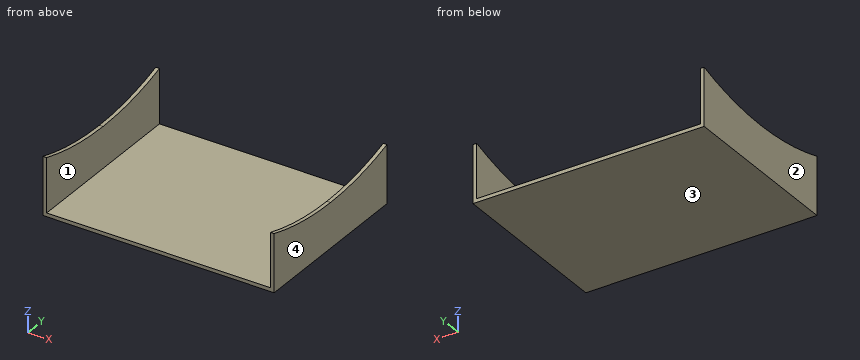
```python
from build123d import *

# Parameters (mm, degrees)
BOSS_EXTRUDE3_DEPTH = 3.18
SKETCH1_5_W         = 3.18
SKETCH1_5_H         = 75
BOSS_EXTRUDE4_DEPTH = 100


with BuildPart() as part:
    # Sketch1 → Boss-Extrude3 (new body)
    with BuildSketch(Plane(origin=(0, 0, 0), x_dir=(0, 0, -1), z_dir=(1, 0, 0))):
        with BuildLine():
            Line((289.494679355, 75), (242.674679355, 75))
            ThreePointArc((242.674679355, 75), (251.152711071, 37.925133117), (254, 0))
            Line((254, 0), (289.494679355, 0))
            Line((289.494679355, 0), (289.494679355, 75))
        make_face()
        with BuildLine():
            Line((289.494679355, 0), (254, 0))
            ThreePointArc((254, 0), (251.152711071, -37.925133117), (242.674679355, -75))
            Line((242.674679355, -75), (289.494679355, -75))
            Line((289.494679355, -75), (289.494679355, 0))
        make_face()
    extrude(amount=BOSS_EXTRUDE3_DEPTH)

    # Sketch1_5 → Boss-Extrude4 (add)
    with BuildSketch(Plane(origin=(0, 0, 0), x_dir=(0, 0, -1), z_dir=(1, 0, 0))):
        with Locations((291.084679355, 37.5)):
            Rectangle(SKETCH1_5_W, SKETCH1_5_H)
        with Locations((291.084679355, -37.5)):
            Rectangle(SKETCH1_5_W, SKETCH1_5_H)
    extrude(amount=BOSS_EXTRUDE4_DEPTH)

    # Mirror2: part across plane


with BuildPart() as part_1:
    add(part.part)
    add(part.part.mirror(Plane(origin=(100, 0, 0), x_dir=(0, 0, 1), z_dir=(1, 0, 0))))


solid = part_1.part
```
Design review of the part built by this model. Coordinates are the model's own, in mm. Face numbers are marked on the shaded views. Round coordinates to 2 decimals unless told otherwise and drop trailing zeros. Order: outer loops, then holes, each group sorted by start corner. A loop starts at its lowest first (then second) coordinate and runs counter-clockwise, first axis right, second up. Notation, with made-up numbers: M 77.25,56 L 82.25,56 A19 ccw 82.25,75 Z; hole C 38.25,-23 d9. An arc over 180 degrees is marked long. Put each result on its own line as item: value.
Q1. Consider section C-C (y = -22). State the section outline as (x, z) points, and give its area (3 significant figures).
Reported:
outline: M 0,-292.67 L 200,-292.67 L 200,-253.05 L 196.82,-253.05 L 196.82,-289.49 L 3.18,-289.49 L 3.18,-253.05 L 0,-253.05 Z
area: 868 mm²
Q2. Consider section D-D (x = 87). State the section outline as (y, z) points, and give its area (3 significant figures).
Reported:
outline: M -75,-292.67 L 75,-292.67 L 75,-289.49 L -75,-289.49 Z
area: 477 mm²
Q3. Insertion check: pin 1 Ø4 at (y, z) = (26.5, -275) entering from -X. The pin has a flat end and moves straight along its axis. Give the tip position at first contact, or say it passes through.
Reported:
pin 1: x = 0
Q4. Draft analysis for pull direction X (two halves, no side actions). For the marked faces 1, 2, 3 and 4, state which applies: released by +X, released by -X, zero draft, split by the parting line, or undercut.
Reported:
face 1: undercut
face 2: released by -X
face 3: zero draft
face 4: released by +X
Q5. To check wall thickness, follow line 1 (X direction, y = 5, z = -260); line 2 (Z direction, x = 10.5, y = -1). State the ranges of each line that lie inside material, in increasing order.
Reported:
line 1: 0 to 3.18, 196.82 to 200
line 2: -292.67 to -289.49
Q6. Consider section A-A (z = -265). State the section outline as (x, y) points, and give its area (3 significant figures).
Reported:
outline: M 0,-75 L 3.18,-75 L 3.18,75 L 0,75 Z; M 196.82,-75 L 200,-75 L 200,75 L 196.82,75 Z
area: 954 mm²
Q7. Consider section B-B (z = -251.5). State the section outline as (x, y) points.
Reported:
outline: M 0,-75 L 3.18,-75 L 3.18,-35.55 L 0,-35.55 Z; M 0,35.55 L 3.18,35.55 L 3.18,75 L 0,75 Z; M 196.82,-75 L 200,-75 L 200,-35.55 L 196.82,-35.55 Z; M 196.82,35.55 L 200,35.55 L 200,75 L 196.82,75 Z
